Input: dimensioned drawing with shaded views. Units: mm. Origin: part minimum x, y, z. Give positions to 0.01 mm unless a question says otherwise; leave off trailing zeros. Order: outer loops, then holes, each group sorted by start corner. A loop starts at its lowest first (then second) coordinate and runs counter-clockwise, first axis right, second up. Notation, with made-up numbers: M 12.5,84 L 45.5,84 A16 ccw 45.5,88 Z; hole C 73,80 d8. An arc over 180 degrees is marked long. Answer in a Markdown table with one row per item. Add a question column.
(1) Material intervals for line 1 along X through (y, z) = (27, 89) (1 decimal); line 2 along Y through (x, z) = (17.5, 98) (1 decimal); line 3 along Y through (x, z) = (37, 113.5) (1 decimal), sorted ascending.
(2) Pin query (flat end, axial travel): P1, Ø6, axis at y = 9.5, z = 46, coming from the +X side; P2, Ø1, axis at x = 29, z = 107.5, coming from the -Y side; P3, Ø8, axis at x = 23, z = 33, coming from the +Y side. Return the tip coordinate at first contact, or that it passes through.
(3) Section query A-A, the plane y = 37. Return loops of the section in (x, z).
(4) Section query B-B, the plane x = 29.5. Return loops of the section in (y, z) (1 decimal), plus the area to 3 significant figures.
(5) Section query D-D, the plane x = 10.5. Return loops of the section in (y, z), plus the area to 3 significant figures.
(6) Mould query, pull axis Y, two halves, no side actions, for the marked faces 1, 2 and 3. Classes: pulls with the +Y half, pulls with the -Y half, needs draft (parallel to the pull), parting line crosses it, or undercut.
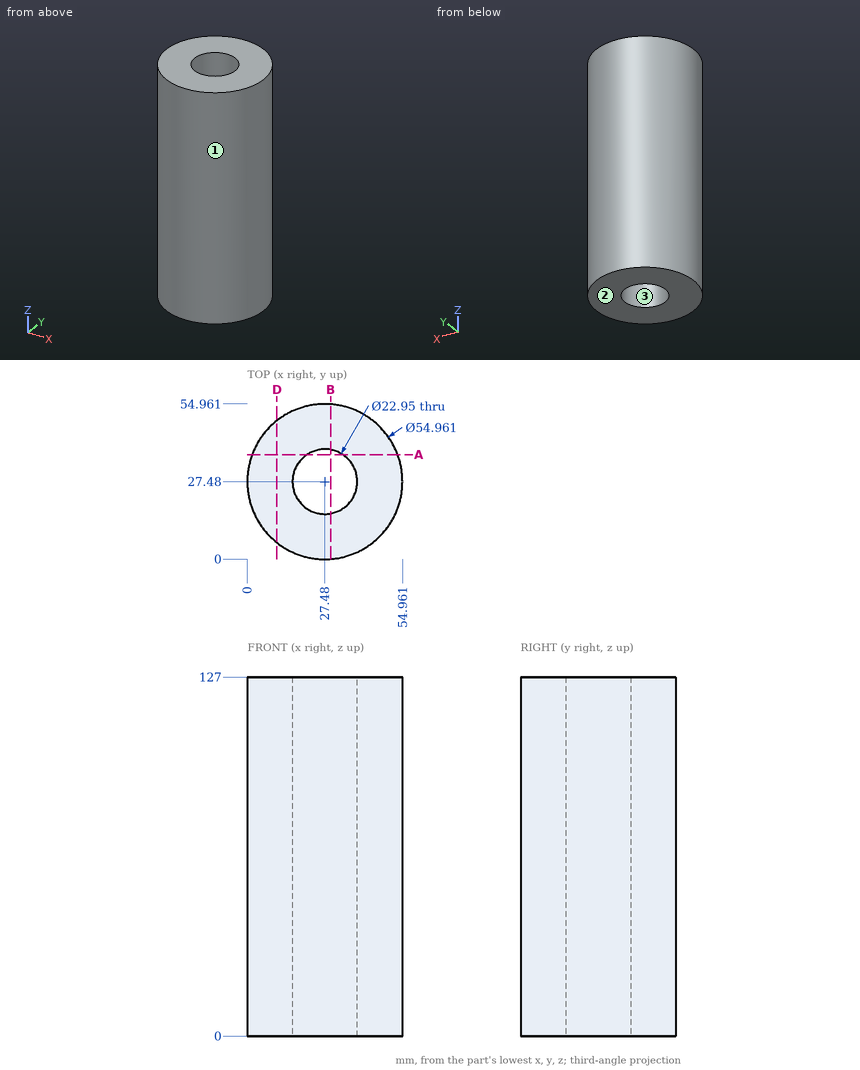
Values follow:
| question | item | result |
|---|---|---|
| 1 | line 1 | x = 0 to 16, 38.9 to 55 |
| 1 | line 2 | y = 1.9 to 21.8, 33.1 to 53.1 |
| 1 | line 3 | y = 1.7 to 21.1, 33.9 to 53.3 |
| 2 | P1 | stops at x = 50.52 |
| 2 | P2 | stops at y = 0.02 |
| 2 | P3 | stops at y = 54.96 |
| 3 | outline | M 1.7,0 L 21.07,0 L 21.07,127 L 1.7,127 Z; M 33.89,0 L 53.26,0 L 53.26,127 L 33.89,127 Z |
| 4 | outline | M 0.1,0 L 16.2,0 L 16.2,127 L 0.1,127 Z; M 38.8,0 L 54.9,0 L 54.9,127 L 38.8,127 Z |
| 4 | area | 4,090 mm² |
| 5 | outline | M 5.87,0 L 49.09,0 L 49.09,127 L 5.87,127 Z |
| 5 | area | 5,490 mm² |
| 6 | face 1 | parting line crosses it |
| 6 | face 2 | needs draft |
| 6 | face 3 | undercut |
